Design review of the part shown in the three views and the two pictorial views. Dimensions are in mm from the part's minimum x, y and z. Round coordinates to 2 decimals unless told otherwise and drop trailing zeros. Loops run counter-clockwise (first coordinate to the right, second up) from the corner with the lowest first, then second, coordinate; pieces in that order, holes last. Notation, with made-up numbers: M -38.5,63.5 L 2.5,63.5 A7 cw 2.5,72.5 Z; hole C 53.5,74.5 d9. An arc over 180 degrees is marked long. Return JSON: item names as keys, results as strings. Group by question number.
Q1. To check wall thickness, follow line 1 along Z through (x, y) = (31, 1.5); line 2 along Y through (x, z) = (5, 3.15); line 3 along X through (y, z) = (1, 2.75). State the ranges of each line that lie inside material, in increasing order.
Q2. Consider section A-A (y = 3.5). State the section outline as (x, z) points.
Q3. Consider section B-B (x = 23). State the section outline as (y, z) points, and give its area (3 significant figures).
Q4. Clearance check with flat-ended pins moving along their axes: pin 1 Ø0.8 at (x, z) = (1.5, 3) entering from +Y; pin 2 Ø2 at (x, y) = (21, 6.5) entering from +Z; pin 3 Ø1.1 at (y, z) = (1.5, 3) entering from +X; pin 4 Ø1 at (x, z) = (27.5, 1.5) entering from -Y. State where each tip first meets the part, or that it passes through.
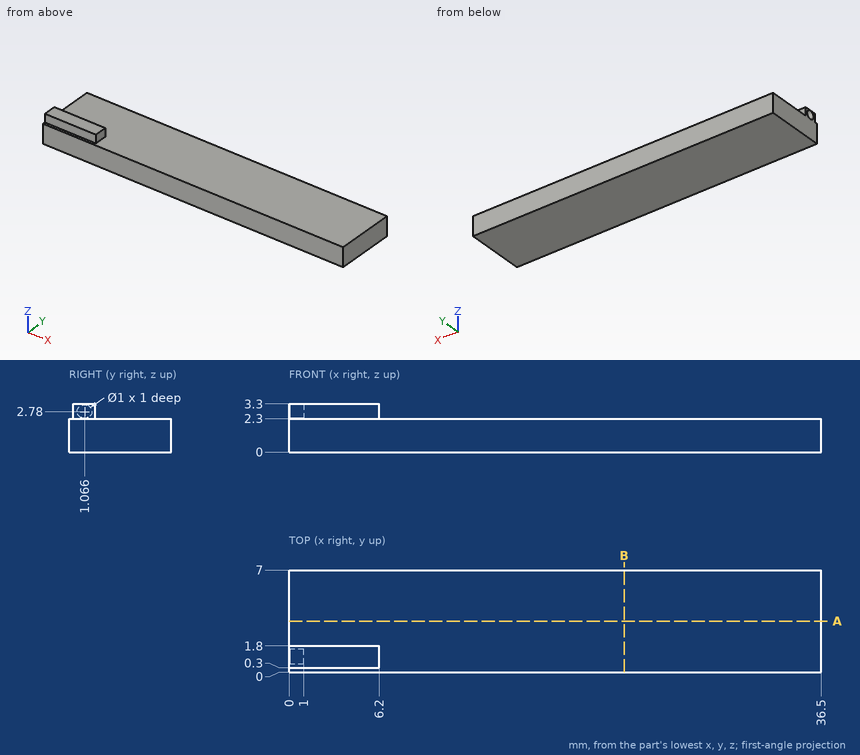
Values:
{
 "1": {"line 1": "z = 0 to 2.3", "line 2": "y = 0.3 to 1.8", "line 3": "x = 1 to 6.2"},
 "2": {"outline": "M 0,0 L 36.5,0 L 36.5,2.3 L 0,2.3 Z"},
 "3": {"outline": "M 0,0 L 7,0 L 7,2.3 L 0,2.3 Z", "area": "16.1 mm2"},
 "4": {"pin 1": "stops at y = 1.8", "pin 2": "stops at z = 2.3", "pin 3": "stops at x = 6.2", "pin 4": "stops at y = 0"}
}
